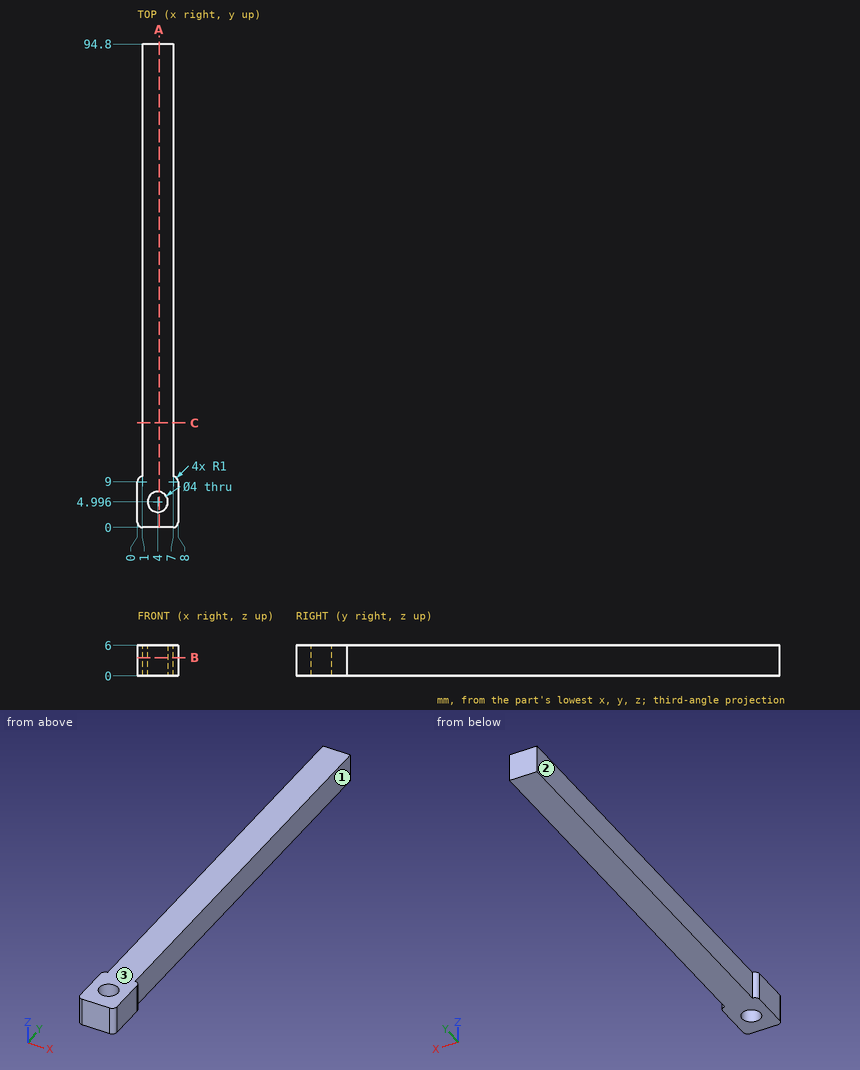
Print and shaded views of the part. All mm, measured from the part's lowest x, y and z. A direction names the side the tool comes from. Coordinates: 2 decimals unless noted, no trailing zeros. Order: outer loops, then holes, each group sorted by start corner. A loop starts at its lowest first (then second) coordinate and runs counter-clockwise, first axis right, second up. Notation, with made-up numbers: M 22,39 L 41,39 A5 cw 41,43 Z; hole C 75.5,80 d9. An arc over 180 degrees is marked long. Answer as CSV lines item,"result".
1) Flat gauge pins, fed straight in: P1, Ø1.8, axis at y = 57.5, z = 2, coming from the +X side; P2, Ø1, axis at y = 13, z = 3.5, coming from the -X side. Where does each tip first touch, or does it go through?
Verdict:
P1,"x = 7"
P2,"x = 1"
2) Cut at B-B (z = 3.6). List the corners of the cut face in (x, y).
Verdict:
outline,"M 0,1 A1 ccw 1,0 L 7,0 A1 ccw 8,1 L 8,9 A1 ccw 7,10 L 7,94.8 L 1,94.8 L 1,10 A1 ccw 0,9 Z; hole C 4,5 d4"
3) 3-axis set-ups, long thin cutter, end or side, ignore diameter. For the marked faces 1, 2 and 3: which of +Z, -Z, +X, -X, +Y, -Y reach the whole face in a straight line?
Verdict:
face 1,"+Z, -Z, +X, +Y"
face 2,"+Z, -Z, -X, +Y"
face 3,"+Z, +X, -X, +Y, -Y"
4) Drill centre lines: L1, parallel to Y at x = 4, z = 1.3; L2, parallel to X at y = 21, z = 4.6; L3, parallel to Y at x = 2.25, z = 3.05. Where is each one in solid material? Low to high. Write a range as from..to.
Verdict:
L1,"0..3, 7..94.8"
L2,"1..7"
L3,"0..4.03, 5.96..94.8"
5) Cut at A-A (x = 4.25). List the corners of the cut face in (y, z).
Verdict:
outline,"M 0,0 L 3.01,0 L 3.01,6 L 0,6 Z; M 6.98,0 L 94.8,0 L 94.8,6 L 6.98,6 Z"
6) Cut at C-C (y = 20.5). List the corners of the cut face in (x, z), then the cut area to 3 significant figures.
Verdict:
outline,"M 1,0 L 7,0 L 7,6 L 1,6 Z"
area,"36.0 mm2"
